```python
from build123d import *

# Parameters (mm, degrees)
F0_W     = 88
F0_H     = 95
F0_R     = 17.5
F1_DEPTH = 12
F2_W     = 88
F2_H     = 12
F3_DEPTH = 38
F5_DEPTH = 12
F7_D     = 4.2
F7_DEPTH = 12
F7_TIP   = 1.2618073
F8_SIZE  = 5


with BuildPart() as f1:
    # F0 (on Front) → F1 (new body)
    with BuildSketch(Plane.XZ):
        with Locations((0, 47.5)):
            Rectangle(F0_W, F0_H)
        with Locations((0, 36)):
            Circle(F0_R, mode=Mode.SUBTRACT)
    extrude(amount=F1_DEPTH)

    # F2 (on face) → F3 (join)
    with BuildSketch(Plane(origin=(0, 0, 0), x_dir=(-1, 0, 0), z_dir=(0, 1, 0))):
        with Locations((0, 6)):
            Rectangle(F2_W, F2_H)
    extrude(amount=F3_DEPTH)

    # F4 (on face) → F5 (cut, through all)
    with BuildSketch(Plane.XY.offset(12)):
        with BuildLine():
            ThreePointArc((26.5, 15), (32, 9.5), (37.5, 15))
            Line((37.5, 15), (37.5, 21))
            ThreePointArc((37.5, 21), (32, 26.5), (26.5, 21))
            Line((26.5, 21), (26.5, 15))
        make_face()
        with BuildLine():
            ThreePointArc((-37.5, 15), (-32, 9.5), (-26.5, 15))
            Line((-26.5, 15), (-26.5, 21))
            ThreePointArc((-26.5, 21), (-32, 26.5), (-37.5, 21))
            Line((-37.5, 21), (-37.5, 15))
        make_face()
    extrude(amount=-F5_DEPTH, mode=Mode.SUBTRACT)

    # F7
    with Locations(Plane.XZ.offset(12)):
        with Locations((-33.2340187158, 84.2340187158), (33.2340187158, 84.2340187158), (33.2340187158, 17.7659812842), (-33.2340187158, 17.7659812842)):
            Hole(F7_D / 2, depth=F7_DEPTH)
            with Locations((0, 0, -(F7_DEPTH + F7_TIP / 2))):  # 118° drill point
                Cone(0, F7_D / 2, F7_TIP, mode=Mode.SUBTRACT)

    # F8
    f8_edges = [f1.edges().sort_by_distance(p)[0] for p in [
        (-44, -6, 95),
        (44, -6, 95),
        (-44, 38, 6),
        (44, 38, 6),
    ]]
    chamfer(f8_edges, length=F8_SIZE)


solid = f1.part
```
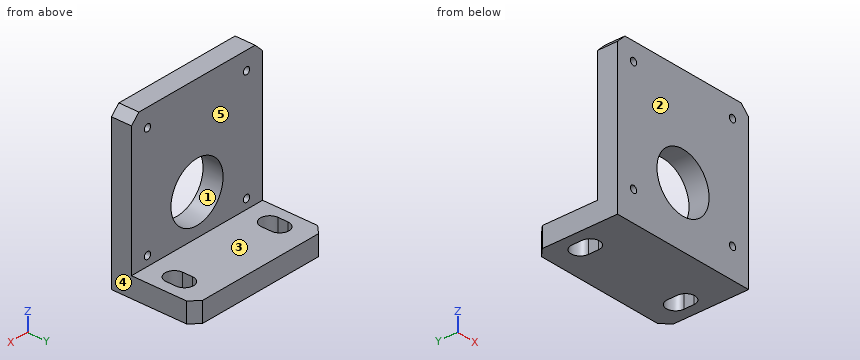
Source: CAD feature listing. Evaluate the final solid. Frame: model axes, mm. Face numbers are marked on the shaded views. A direction names the side the tool comes from. Give positions to 0.01 mm unless a question says otherwise; leave off trailing zeros. Loops run counter-clockwise (first coordinate to the right, second up) from the corner with the lowest first, then second, coordinate; pieces in that order, holes last. Notation, with made-up numbers: M 79,-8.5 L 114,-8.5 A23 cw 114,10.5 Z; hole C -0.75,50.25 d3. An arc over 180 degrees is marked long. Put each result on its own line as item: value.
Q1. Section B-B (x = 0). Return the cut outline in (y, z), and give its area (3 significant figures).
Response values:
outline: M -12,0 L 38,0 L 38,12 L 0,12 L 0,18.5 L -12,18.5 Z; M -12,53.5 L 0,53.5 L 0,95 L -12,95 Z
area: 1,180 mm²
Q2. Section A-A (z = 36). Return the cut outline in (x, y), and give its area (3 significant figures).
Response values:
outline: M -44,-12 L -17.5,-12 L -17.5,0 L -44,0 Z; M 17.5,-12 L 44,-12 L 44,0 L 17.5,0 Z
area: 636 mm²
Q3. Reachability of the marked faces 4 and 5 from +Z, -Z, +X, -X, +Y, -Y: full face, straight path, thin tool, end or side. Return the list, or none.
Response values:
face 4: +Z, -Z, +X, +Y, -Y
face 5: +Z, +X, -X, +Y
Q4. Section D-D (y = -2). Return the cut outline in (x, z).
Response values:
outline: M -44,0 L 44,0 L 44,90 L 39,95 L -39,95 L -44,90 Z; hole C -33.23,17.77 d4.2; hole C -33.23,84.23 d4.2; hole C 0,36 d35; hole C 33.23,17.77 d4.2; hole C 33.23,84.23 d4.2
Q5. Line query: probe 1 along Y at (x, z) = (-31.5, 8); probe 2 along Z at (x, y) = (0, -8); probe 3 along Y at (x, z) = (-21, 64). Output: solid intervals per line, ascending. Write a range as [from, to].
Response values:
probe 1: y = [-12, 9.52], [26.48, 38]
probe 2: z = [0, 18.5], [53.5, 95]
probe 3: y = [-12, 0]
Q6. Pin query (flat end, axial travel): P1, Ø1, axis at x = -13, z = 20, coming from the +Y side; P2, Ø3, axis at x = 20.5, y = 15, coming from the +Z side; P3, Ø2.5, axis at x = -33.23, z = 17.77, coming from the +Y side. Return the tip coordinate at first contact, or that it passes through.
Response values:
P1: stops at y = 0
P2: stops at z = 12
P3: passes through
Q7. Section C-C (z = 8). Return the cut outline in (x, y).
Response values:
outline: M -44,-12 L 44,-12 L 44,33 L 39,38 L -39,38 L -44,33 Z; hole M -37.5,15 A5.5 ccw -26.5,15 L -26.5,21 A5.5 ccw -37.5,21 Z; hole M 26.5,15 A5.5 ccw 37.5,15 L 37.5,21 A5.5 ccw 26.5,21 Z
Q8. Mould query, pull axis Z, two halves, no side actions, for the marked faces 1, 2 and 3. Classes: released by +Z, released by -Z, zero draft, split by the parting line, or undercut.
Response values:
face 1: undercut
face 2: zero draft
face 3: released by +Z
